Read the model definition and answer for the solid it produces. Units are mm, in the model's axes. A direction names the side the tool comes from. Give positions to 0.01 mm unless a question says otherwise; leave off trailing zeros. Order: outer loops, then holes, each group sorted by start corner. A loop starts at its lowest first (then second) coordinate and runs counter-clockwise, first axis right, second up.
```python
from build123d import *

# Parameters (mm, degrees)
F0_R     = 3.625
F1_DEPTH = 2.75
F2_T     = -1.25
F4_DEPTH = 1.5
F5_R     = 3.5
F6_DEPTH = 0.5
F8_R     = 0.1


# Not quite as in the source:
# - a fillet or chamfer that OpenCascade refuses, or shapes differently, is made with other operations: its cross-section is extruded or revolved along the edge and cut away or added


with BuildPart() as f1:
    # F0 (on Right) → F1 (new body, symmetric)
    with BuildSketch(Plane.YZ):
        Circle(F0_R)
    extrude(amount=F1_DEPTH, both=True)

    # F2
    f2_openings = [f1.faces().sort_by_distance(p)[0] for p in [
        (-2.75, 0, 0),
    ]]
    offset(amount=F2_T, openings=f2_openings)

    # F3 (on face) → F4 (join)
    with BuildSketch(Plane(origin=(-2.75, 0, 0), x_dir=(0, -1, 0), z_dir=(-1, 0, 0))):
        with BuildLine():
            Line((3.5465652398, -0.75), (5.0465652398, -0.75))
            Line((5.0465652398, -0.75), (5.0465652398, 0.75))
            Line((5.0465652398, 0.75), (3.5465652398, 0.75))
            ThreePointArc((3.5465652398, 0.75), (3.625, 0), (3.5465652398, -0.75))
        make_face()
        with BuildLine():
            Line((-3.5465652398, 0.75), (-5.0465652398, 0.75))
            Line((-5.0465652398, 0.75), (-5.0465652398, -0.75))
            Line((-5.0465652398, -0.75), (-3.5465652398, -0.75))
            ThreePointArc((-3.5465652398, -0.75), (-3.625, 0), (-3.5465652398, 0.75))
        make_face()
    extrude(amount=-F4_DEPTH)

    # F5 (on face) → F6 (cut)
    with BuildSketch(Plane.YZ.offset(2.75)):
        Circle(F5_R)
    extrude(amount=-F6_DEPTH, mode=Mode.SUBTRACT)

    # F7: fillet of radius 9 on 1 edges, made by hand

    # F7_s1 → F7_t2 (revolve)
    with BuildSketch(Plane.XY):
        with BuildLine():
            ThreePointArc((2.75, 3.5), (2.3758803254, 2.0419601084), (2.25, 0.5419601084))
            Line((2.25, 0.5419601084), (2.25, 3.5))
            Line((2.25, 3.5), (2.75, 3.5))
        make_face()
    revolve(axis=Axis((2.25, 0, 0), (1, 0, 0)))

    # F8
    f8_edges = [f1.edges().sort_by_distance(p)[0] for p in [
        (2.75, -3.5, 0),
        (2.75, -3.625, 0),
    ]]
    fillet(f8_edges, radius=F8_R)


solid = f1.part
```
1) The part is cut by section B-B on x = 0.55. Determine the outline of the cut face in (y, z) (3 decimals), and give its area (3 significant figures).
Final values:
outline: circle Ø7.25 at (0, 0); hole circle Ø4.75 at (0, 0)
area: 23.6 mm2
2) For a pull along Z with two mould halves and no side action, classify faces 1 (the face through (-2, -5.047, 0)), 2 (the face through (-0.595, 1.096, -2.107)), 3 (the face through (2.25, 0, 0)), 4 (the face through (-0.012, 3.458, 1.089)) as released by +Z, released by -Z, zero draft, split by the parting line, or undercut.
Final values:
face 1: zero draft
face 2: undercut
face 3: undercut
face 4: split by the parting line
3) Given pin 1 (0.9 mm diameter, centred on y = 0, z = 0, fed in from +X); pin 2 (1 mm diameter, centred on x = 1.5, y = -3, fed in from -Z) (3 decimals); pin 3 (1.2 mm diameter, centred on y = -4.5, z = 0, fed in from +X); pin 4 (3 mm diameter, centred on x = -0.5, z = 0.5, fed in from +Y), each flat-ended and moving along its own axis, determine where each tip first touches the part or whether it passes through.
Final values:
pin 1: stops at x = 2.25
pin 2: stops at z = -2.625
pin 3: stops at x = -1.25
pin 4: stops at y = 5.05
4) Consider L1, parallel to Z at x = -1.7, y = 0 (3 decimals); L2, parallel to Z at x = -0.75, y = 0.75; L3, parallel to Y at x = 1.3, z = -0.25. Determine where each line is inside the solid, lowest interval first.
Final values:
L1: z = -3.625 to -2.375, 2.375 to 3.625
L2: z = -3.55 to -2.25, 2.25 to 3.55
L3: y = -3.62 to -2.36, 2.36 to 3.62
5) The part is cut by section A-A on y = -4.5. Determine the outline of the cut face in (x, z).
Final values:
outline: (-2.75, -0.75) - (-1.25, -0.75) - (-1.25, 0.75) - (-2.75, 0.75) - close
6) A tool of negligible diameter and unlimited length cuts with its end or side. For faces 5 (the face through (-2, 4, 0.75)), 6 (the face through (-2, -4, -0.75)), 7 (the face through (-2, 4, -0.75)), from which of +Z, -Z, +X, -X, +Y, -Y can it reach the whole face along a straight path? Write none if from no direction.
Final values:
face 5: +Z, +X, -X, +Y
face 6: -Z, +X, -X, -Y
face 7: -Z, +X, -X, +Y
